CAD build for the part. Positions are in the model's coordinates, mm. Coordinates: 2 decimals unless noted, no trailing zeros. Loops run counter-clockwise (first coordinate to the right, second up) from the corner with the lowest first, then second, coordinate; pieces in that order, holes last.
1) Pin check, flat tips, straight feed: pin 1 Ø2 at (x, y) = (3, 177.78) entering from -Z; pin 2 Ø1.8 at (y, z) = (44.5, 4) entering from -X. Stop position of each tip, or through.
2) Wall check: line 1 along Y through (x, z) = (487, 3.25); line 2 along X through (y, z) = (56.5, 5.4). Give the ranges that are in metal, low to high.
3) Saw through at A-A, the plane z = 3.3. Write the cut outline in (x, y).
```python
from build123d import *

# Parameters (mm, degrees)
SKETCH1_W            = 490
SKETCH1_H            = 400
BOSS_EXTRUDE1_DEPTH  = 6
SKETCH2_W            = 6
SKETCH2_H            = 133.333333333
CUT_EXTRUDE1_DEPTH   = 12
M3_CLEARANCE_HOLE1_D = 3.4


with BuildPart() as part:
    # Sketch1 → Boss-Extrude1 (new body)
    with BuildSketch(Plane.XY):
        with Locations((245, 200)):
            Rectangle(SKETCH1_W, SKETCH1_H)
    extrude(amount=BOSS_EXTRUDE1_DEPTH)

    # Sketch2 → Cut-Extrude1 (cut)
    with BuildSketch(Plane.XY.offset(6)):
        with Locations((487, 333.333333334)):
            Rectangle(SKETCH2_W, SKETCH2_H)
        with Locations((3, 333.333333334)):
            Rectangle(SKETCH2_W, SKETCH2_H)
        with Locations((3, 66.666666667)):
            Rectangle(SKETCH2_W, SKETCH2_H)
        with Locations((487, 66.666666667)):
            Rectangle(SKETCH2_W, SKETCH2_H)
    extrude(amount=-CUT_EXTRUDE1_DEPTH, mode=Mode.SUBTRACT)

    # M3 Clearance Hole1 (through all)
    with Locations(Plane.XY.offset(6)):
        with Locations((3, 222.223333333), (3, 177.776666667), (487, 222.223333333), (487, 177.776666667)):
            Hole(M3_CLEARANCE_HOLE1_D / 2)


solid = part.part
```
Data:
1. pin 1: passes through
1. pin 2: stops at x = 6
2. line 1: y = 133.33 to 176.08, 179.48 to 220.52, 223.92 to 266.67
2. line 2: x = 6 to 484
3. outline: (0, 133.33) - (6, 133.33) - (6, 0) - (484, 0) - (484, 133.33) - (490, 133.33) - (490, 266.67) - (484, 266.67) - (484, 400) - (6, 400) - (6, 266.67) - (0, 266.67) - close; hole circle Ø3.4 at (3, 177.78); hole circle Ø3.4 at (3, 222.22); hole circle Ø3.4 at (487, 177.78); hole circle Ø3.4 at (487, 222.22)
